Here's the drawing with two shaded views (mm, measured from the low corner). I have some questions. Give positions to 0.01 mm unless a question says otherwise; leave off trailing zeros. Write each loop counter-clockwise with the first axis right and the second up, starting at its lowest first coordinate (ties: lowest second). Pieces come first, ordered by that corner, then holes. Notation, with made-up numbers: M 55.25,76.25 L 113.25,76.25 A11 cw 113.25,80.25 Z; hole C 38,-21 d1. An arc over 180 degrees is marked long. Use one line per item in the form item = value. Start each with the question number.
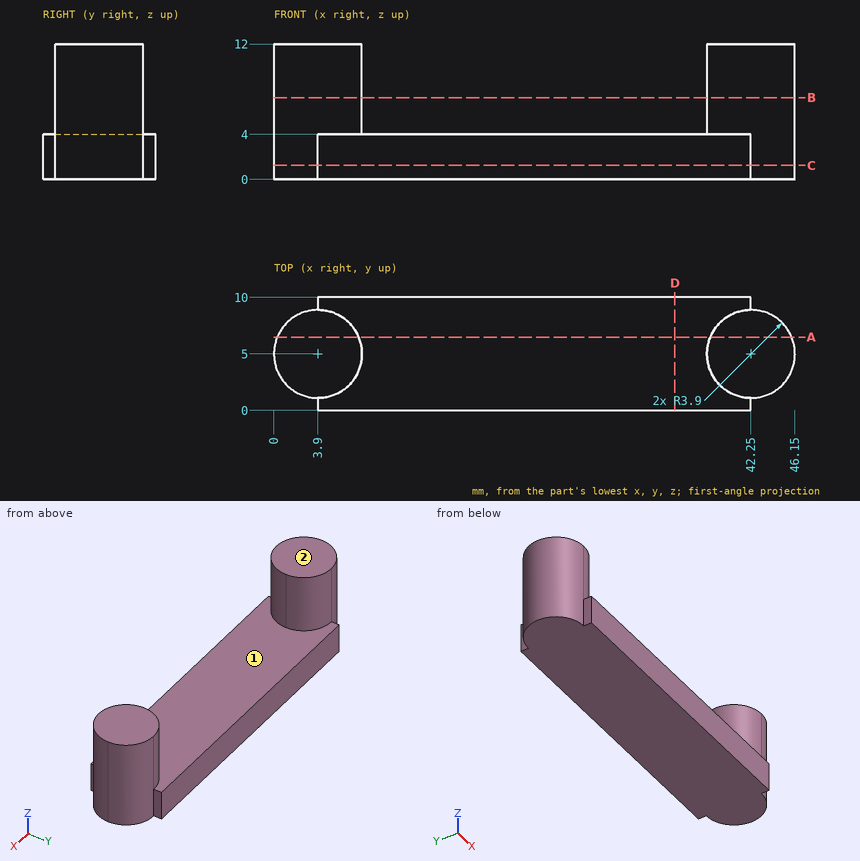
1) Suppose I cut it at B-B, the plane z = 7.25. List the corners of the cut face in (x, y) for me.
2) Suppose I cut it at C-C, the plane z = 1.25. List the corners of the cut face in (x, y) for me.
3) Will these pins go through, and if not, where does the flat tip stop? P1, Ø0.5, axis at y = 9.5, z = 2.5, coming from the +X side; P2, Ø6, axis at y = 3, z = 4, coming from the -X side; P3, Ø0.6, axis at y = 0.5, z = 1, coming from the -X side; P4, Ø3, axis at x = 27, y = 6.5, coming from the +Z side.
4) Please list where these lines run through material, in increasing order: line 1 (Z direction, x = 34, y = 3.5); line 2 (X direction, y = 6, z = 4.75); line 3 (X direction, y = 2.25, z = 7.5).
5) Thinking about a two-plate mould opening in X: for the marked faces 1 and 2, which applies, released by +X, released by -X, zero draft, split by the parting line, or undercut?
6) Suppose I cut it at D-D, the plane x = 35.5. List the corners of the cut face in (y, z) for me.
7) Suppose I cut it at A-A, the plane y = 6.5. List the corners of the cut face in (x, z) for me.
Checks:
q1.outline = C 3.9,5 d7.8; C 42.25,5 d7.8
q2.outline = M 3.9,0 L 42.25,0 L 42.25,1.1 A3.9 ccw 42.25,8.9 L 42.25,10 L 3.9,10 L 3.9,8.9 A3.9 ccw 3.9,1.1 Z
q3.P1 = 42.25
q3.P2 = 0
q3.P3 = 3.9
q3.P4 = 4
q4.line_1 = 0 to 4
q4.line_2 = 0.13 to 7.67, 38.48 to 46.02
q4.line_3 = 1.13 to 6.67, 39.48 to 45.02
q5.face_1 = undercut
q5.face_2 = zero draft
q6.outline = M 0,0 L 10,0 L 10,4 L 0,4 Z
q7.outline = M 0.3,0 L 45.85,0 L 45.85,12 L 38.65,12 L 38.65,4 L 7.5,4 L 7.5,12 L 0.3,12 Z
